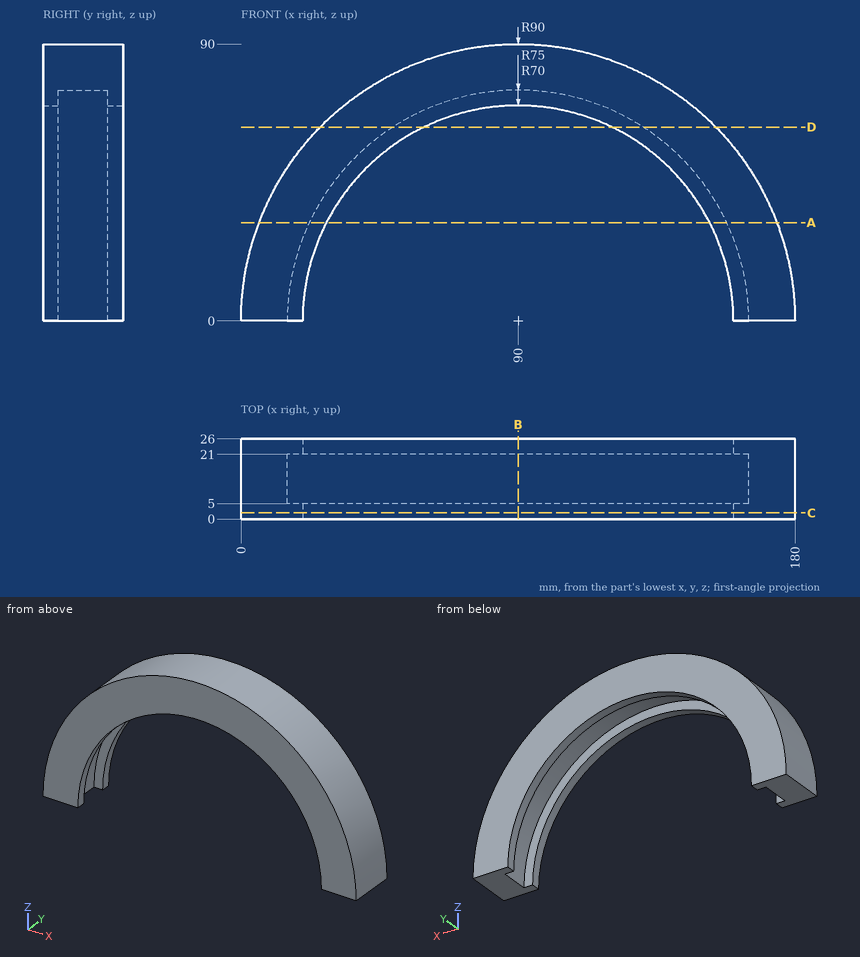
Can you work these out from the drawing? Everything is in mm from the part's minimum corner. Round coordinates to 2 decimals unless told otherwise and drop trailing zeros. Loops run counter-clockwise (first coordinate to the right, second up) from the corner with the lowest first, then second, coordinate; pieces in that order, holes last. Notation, with made-up numbers: (70, -8) -> (105, -8) arc R17 ccw to (105, 19) -> close; hole circle Ø10 at (-29.5, 14). An arc over 180 degrees is marked (long way). Use CSV: the item, a comma, the result in double quotes.
(1) Suppose I cut it at A-A on z = 32. Write out the boundary of the cut face in (x, y), plus the area to 3 significant figures.
Return value:
outline,"(5.88, 0) -> (27.74, 0) -> (27.74, 5) -> (22.17, 5) -> (22.17, 21) -> (27.74, 21) -> (27.74, 26) -> (5.88, 26) -> close; (152.26, 0) -> (174.12, 0) -> (174.12, 26) -> (152.26, 26) -> (152.26, 21) -> (157.83, 21) -> (157.83, 5) -> (152.26, 5) -> close"
area,"958 mm²"
(2) Will these pins go through, and if not, where does the flat tip stop? pin 1 Ø3 at (x, y) = (125.5, 5.5) entering from +Z; pin 2 Ø10 at (x, y) = (24, 7) entering from +Z; pin 3 Ø4 at (x, y) = (111, 3.5) entering from -Z; pin 4 Ø22.5 at (x, z) = (67, 52) entering from -Y.
Return value:
pin 1,"stops at z = 83.33"
pin 2,"stops at z = 66.17"
pin 3,"stops at z = 66.11"
pin 4,"passes through"
(3) Suppose I cut it at B-B on x = 90. Write out the boundary of the cut face in (y, z), plus the area to 3 significant figures.
Return value:
outline,"(0, 70) -> (5, 70) -> (5, 75) -> (21, 75) -> (21, 70) -> (26, 70) -> (26, 90) -> (0, 90) -> close"
area,"440 mm²"
(4) If I drill on probe 1 along Y at (x, z) = (78.5, 73.5); probe 2 along X at (y, z) = (8.75, 54); probe 3 along X at (y, z) = (7, 44), over which ranges is the centre line in solid material (lowest first)? Write a range as [from, to].
Return value:
probe 1,"y = [0, 5], [21, 26]"
probe 2,"x = [18, 37.95], [142.05, 162]"
probe 3,"x = [11.49, 29.26], [150.74, 168.51]"
(5) Suppose I cut it at C-C on y = 2. Write out the boundary of the cut face in (x, z).
Return value:
outline,"(0, 0) -> (20, 0) arc R70 cw to (160, 0) -> (180, 0) arc R90 ccw to start"
(6) Suppose I cut it at D-D on z = 63. Write out the boundary of the cut face in (x, y).
Return value:
outline,"(25.73, 0) -> (59.49, 0) -> (59.49, 5) -> (49.31, 5) -> (49.31, 21) -> (59.49, 21) -> (59.49, 26) -> (25.73, 26) -> close; (120.51, 0) -> (154.27, 0) -> (154.27, 26) -> (120.51, 26) -> (120.51, 21) -> (130.69, 21) -> (130.69, 5) -> (120.51, 5) -> close"
